Autodesk Fusion 360 part; units mm, degrees
sketch "Sketch1" plane through (0, 0, 0) normal (0, 0, 1) x (1, 0, 0)
  line L0 (0, 0) -> (10, 0)
  line L1 (10, 0) -> (10, 10)
  line L2 (10, 10) -> (0, 10)
  line L3 (0, 10) -> (0, 0)
  line L4 (0, 10) -> (10, 0)
  line L5 (0, 0) -> (10, 10)
  circle A0 centre (5, 5) radius 2
  dimension "d1" = 10
  dimension "d2" = 10
  dimension "d3" = 4
extrude "Extrude1" add sketch "Sketch1" along normal blind 2.5 contours L0 L4 L5 A0 | L3 L4 L5 A0 | L1 L4 L5 A0 | L2 L4 L5 A0
sketch "Sketch2" plane through (0, 0, 2.5) normal (0, 0, 1) x (-1, 0, 0)
  circle A0 centre (-5, -5) radius 2
  line L0 (0, -10) -> (0, 0)
  line L1 (0, 0) -> (-10, 0)
  line L2 (-10, 0) -> (-10, -10)
  line L3 (-10, -10) -> (0, -10)
  line L4 (0, 0) -> (-10, 0)
  line L5 (-10, 0) -> (-10, 2)
  line L6 (-10, 2) -> (0, 2)
  line L7 (0, 2) -> (0, 0)
  line L8 (0, 0) -> (-10, 0)
  line L9 (-10, 0) -> (-10, 1.5)
  line L10 (-10, 1.5) -> (0, 1.5)
  line L11 (0, 1.5) -> (0, 0)
  line L12 (-5, 0) -> (3, 0)
  line L13 (3, 0) -> (3, 1.5)
  line L14 (3, 1.5) -> (-5, 1.5)
  line L15 (-5, 1.5) -> (-5, 0)
  line L16 (-5, 0) -> (-13, 0)
  line L17 (-13, 0) -> (-13, 1.5)
  line L18 (-13, 1.5) -> (-5, 1.5)
  line L19 (-5, 1.5) -> (-5, 0)
  line L20 (3, 0) -> (1.5, 0)
  line L21 (1.5, 0) -> (1.5, 1.5)
  line L22 (1.5, 1.5) -> (3, 1.5)
  line L23 (3, 1.5) -> (3, 0)
  line L24 (3, 0) -> (1.5, 0)
  line L25 (1.5, 0) -> (1.5, 20)
  line L26 (1.5, 20) -> (3, 20)
  line L27 (3, 20) -> (3, 0)
  line L28 (-13, 0) -> (-11.5, 0)
  line L29 (-11.5, 0) -> (-11.5, 20)
  line L30 (-11.5, 20) -> (-13, 20)
  line L31 (-13, 20) -> (-13, 0)
  line L32 (1.5, 20) -> (0, 20)
  line L33 (0, 20) -> (0, 18.5)
  line L34 (0, 18.5) -> (1.5, 18.5)
  line L35 (1.5, 18.5) -> (1.5, 20)
  line L36 (-11.5, 20) -> (-10, 20)
  line L37 (-10, 20) -> (-10, 18.5)
  line L38 (-10, 18.5) -> (-11.5, 18.5)
  line L39 (-11.5, 18.5) -> (-11.5, 20)
  line L40 (1.5, 2) -> (-11.5, 2)
  line L41 (-11.5, 2) -> (-11.5, 18.5)
  line L42 (-11.5, 18.5) -> (1.5, 18.5)
  line L43 (1.5, 18.5) -> (1.5, 2)
  line L44 (1.5, 0) -> (0, -1.5)
  line L45 (1.5, 0) -> (3.6213, 0) construction
  line L46 (-11.5, 0) -> (-10, -1.5)
  dimension "d6" = 2
  dimension "d7" = 1.5
  dimension "d8" = 8
  dimension "d9" = 20
  dimension "d10" = 1.5
  dimension "d11" = 20
  dimension "d12" = 1.5
  dimension "d13" = 1.5
  dimension "d14" = 1.5
  dimension "d15" = 1.5
  dimension "d16" = 135
  dimension "d17" = 90
extrude "Extrude2" add sketch "Sketch2" along normal blind 2 contours L0 L1 L2 L3 L4 L8 L12 L16 | L0 L12 L44 | L1 L4 L7 L8 L10 L11 L12 L14 L15 L19 | L7 L11 L12 L14 L21 L25 | L2 L16 L46 | L1 L4 L5 L8 L9 L10 L15 L16 L18 L19 | L5 L6 L7 L10 L14 L18 L40 | L7 L14 L25 L40 | L5 L9 L16 L18 L29 | L6 L25 L29 L34 L38 L40 L41 L42 L43 | L5 L18 L29 L40
sketch "Sketch3" plane through (0, 0, 2.5) normal (0, 0, -1) x (1, 0, 0)
  line L0 (10, 0) -> (10, -1.5)
  line L1 (10, -1.5) -> (11.5, 0)
  line L2 (11.5, 0) -> (11.5, 18.5)
  line L3 (11.5, 18.5) -> (-1.5, 18.5)
  line L4 (-1.5, 18.5) -> (-1.5, 0)
  line L5 (-1.5, 0) -> (0, -1.5)
  line L6 (0, -1.5) -> (0, 0)
  line L7 (0, 0) -> (10, 0)
  line L8 (-1.5, 0) -> (11.5, 0)
  line L9 (11.5, 0) -> (11.5, -1.5)
  line L10 (11.5, -1.5) -> (-1.5, -1.5)
  line L11 (-1.5, -1.5) -> (-1.5, 0)
  line L12 (-1.5, 0) -> (11.5, 0)
  line L13 (11.5, 0) -> (11.5, 2)
  line L14 (11.5, 2) -> (-1.5, 2)
  line L15 (-1.5, 2) -> (-1.5, 0)
  line L16 (-1.5, 18.5) -> (-1, 18.5)
  line L17 (-1, 2) -> (-1.5, 2)
  line L18 (-1.5, 2) -> (-1.5, 18.5)
  line L19 (11.5, 18.5) -> (11, 18.5)
  line L20 (11, 2) -> (11.5, 2)
  line L21 (11.5, 2) -> (11.5, 18.5)
  line L22 (-1.5, 18.5) -> (0, 18.5)
  line L23 (0, 18.5) -> (0, 20)
  line L24 (0, 20) -> (-1.5, 20)
  line L25 (-1.5, 20) -> (-1.5, 18.5)
  line L26 (11.5, 18.5) -> (10, 18.5)
  line L27 (10, 18.5) -> (10, 20)
  line L28 (10, 20) -> (11.5, 20)
  line L29 (11.5, 20) -> (11.5, 18.5)
  line L30 (10, 20) -> (9.75, 20)
  line L31 (9.75, 20) -> (9.75, 18.5)
  line L32 (9.75, 18.5) -> (10, 18.5)
  line L33 (10, 18.5) -> (10, 20)
  line L34 (0, 20) -> (0.25, 20)
  line L35 (0.25, 20) -> (0.25, 18.5)
  line L36 (0.25, 18.5) -> (0, 18.5)
  line L37 (0, 18.5) -> (0, 20)
  line L38 (-1.5, 20) -> (-1.25, 20)
  line L39 (-1.25, 20) -> (-1.25, 2)
  line L40 (-1.25, 2) -> (-1.5, 2)
  line L41 (-1.5, 2) -> (-1.5, 20)
  line L42 (11.5, 2) -> (11.25, 2)
  line L43 (11.25, 2) -> (11.25, 18.5)
  line L44 (11.25, 18.5) -> (11.5, 18.5)
  line L45 (11.5, 18.5) -> (11.5, 2)
  line L46 (-1.5, 18.5) -> (0.25, 18.5)
  line L47 (0.25, 18.5) -> (0.25, 18.25)
  line L48 (0.25, 18.25) -> (-1.5, 18.25)
  line L49 (-1.5, 18.25) -> (-1.5, 18.5)
  line L50 (9.75, 18.5) -> (11.25, 18.5)
  line L51 (11.25, 18.5) -> (11.25, 18.25)
  line L52 (11.25, 18.25) -> (9.75, 18.25)
  line L53 (9.75, 18.25) -> (9.75, 18.5)
  line L54 (0.25, 20) -> (9.75, 20)
  line L55 (9.75, 20) -> (9.75, 18.5)
  line L56 (9.75, 18.5) -> (0.25, 18.5)
  line L57 (0.25, 18.5) -> (0.25, 20)
  dimension "d20" = 13
  dimension "d21" = 2
  dimension "d22" = 0.5
  dimension "d23" = 0.5
  dimension "d24" = 1.5
  dimension "d25" = 1.5
  dimension "d26" = 1.5
  dimension "d27" = 1.5
  dimension "d28" = 0.25
  dimension "d29" = 0.25
  dimension "d30" = 0.25
  dimension "d31" = 0.25
  dimension "d32" = 0.25
  dimension "d33" = 0.25
extrude "Extrude3" add sketch "Sketch3" along normal blind 1 contours L3 L14 L17 L20 L39 L43 L47 L48 L52 L53 L56 | L3 L31 L35 L54 L55 L56 L57
sketch "Sketch4" plane through (0, 0, 1.5) normal (0, 0, -1) x (1, 0, 0)
  line L0 (0.25, 18.25) -> (-1.25, 18.25)
  line L1 (-1.25, 18.25) -> (-1.25, 2)
  line L2 (-1.25, 2) -> (11.25, 2)
  line L3 (11.25, 2) -> (11.25, 18.25)
  line L4 (11.25, 18.25) -> (9.75, 18.25)
  line L5 (9.75, 18.25) -> (9.75, 20)
  line L6 (9.75, 20) -> (0.25, 20)
  line L7 (0.25, 20) -> (0.25, 18.25)
  line L8 (0.25, 20) -> (9.75, 20)
  line L9 (9.75, 20) -> (9.75, 18.5)
  line L10 (9.75, 18.5) -> (0.25, 18.5)
  line L11 (0.25, 18.5) -> (0.25, 20)
  dimension "d36" = 1.5
extrude "Extrude4" add sketch "Sketch4" along normal blind 0.5 contours L5 L6 L7 L8 L9 L10 L11
extrude "Extrude5" add 1 faces at (3.4167, -19, 2.5) along direction (0, 0, 1) blind 2
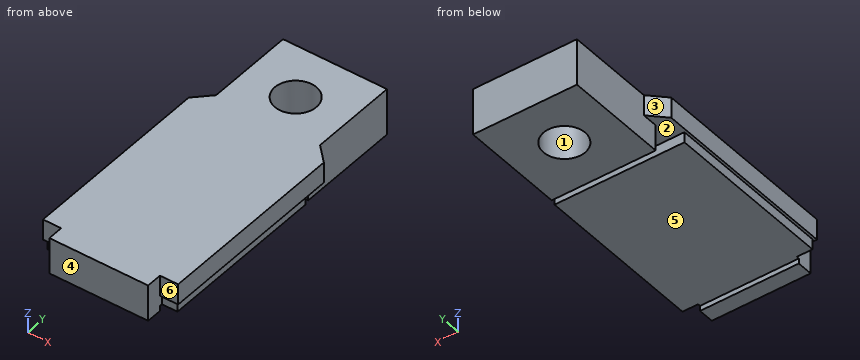
The listing builds one solid part. Answer for the finished solid, in the listing's coordinates (mm). Face numbers are marked on the shaded views. A direction names the side the tool comes from. Round coordinates to 2 decimals unless told otherwise and drop trailing zeros. Write each loop counter-clockwise with the first axis right and the second up, starting at its lowest first coordinate (ties: lowest second). Pieces come first, ordered by that corner, then holes. Notation, with made-up numbers: (-31, 28.25) - (21, 28.25) arc R32 ccw to (21, 54.25) - close; hole circle Ø6 at (10, -15.5). An arc over 180 degrees is marked (long way). Use a Markdown table: item, result. Add a question column.
1. Consider line 1 (Y direction, x = 5, z = 1.4); line 2 (Y direction, x = 5, z = 1.85); line 3 (X direction, y = 5, z = 2.65). Determine where each line is inside the solid, lowest interval first.
2. The part is cut by section A-A (z = 1.95). Write down the section's boundary in (x, y), and give its area (3 significant figures).
3. The part is cut by section B-B (x = 9). Write down the section's boundary in (y, z), and give its area (3 significant figures).
4. A tool of negligible diameter and unlimited length cuts with its end or side. For the marked faces 4, 5 and 6, from which of +Z, -Z, +X, -X, +Y, -Y can it reach the whole face along a straight path? Write none if from no direction.
5. Flat-ended cylindrical pins translate along their axes: P1, Ø1.5, axis at y = 6.5, z = 1.5, coming from the +X side; P2, Ø6.5, axis at x = 2, y = -12.5, coming from the -Z side; P3, Ø0.8, axis at x = 6.5, y = -19.5, coming from the -Z side; P4, Ø0.9, axis at x = 0, z = 4, coming from the -Y side. Find the tip coordinate at first contact, or state that the pin passes through.
6. For a pull along X with two mould halves and no side action, classify the marked faces 1, 2 and 3 as +X half, -X half, draft (parallel to the pull), parting line (faces both ways), or undercut.
7. The part is cut by section C-C (y = -10.75). Write down the section's boundary in (x, z).
Reported:
| question | item | result |
|---|---|---|
| 1 | line 1 | -20 to -18.5, 0 to 3, 7 to 10 |
| 1 | line 2 | -20 to -2, 0 to 3, 7 to 10 |
| 1 | line 3 | 0 to 3, 7 to 10 |
| 2 | outline | (-1.25, -18.25) - (0.25, -18.25) - (0.25, -20) - (9.75, -20) - (9.75, -18.25) - (11.25, -18.25) - (11.25, -2) - (-1.25, -2) - close; (0, 0) - (10, 0) - (10, 10) - (0, 10) - close; hole circle Ø4 at (5, 5) |
| 2 | area | 307 mm^2 |
| 3 | outline | (-20, 1) - (-18.5, 1) - (-18.5, 1.5) - (-2, 1.5) - (-2, 2.5) - (0, 2.5) - (0, 0) - (10, 0) - (10, 4.5) - (-20, 4.5) - close |
| 3 | area | 104 mm^2 |
| 4 | face 4 | +Z, -Z, +X, -X, -Y |
| 4 | face 5 | -Z, +X, -X |
| 4 | face 6 | +Z, -Z, +X, -Y |
| 5 | P1 | x = 10 |
| 5 | P2 | z = 1.5 |
| 5 | P3 | z = 1 |
| 5 | P4 | y = -20 |
| 6 | face 1 | undercut |
| 6 | face 2 | draft |
| 6 | face 3 | -X half |
| 7 | outline | (-1.5, 2.5) - (-1.25, 2.5) - (-1.25, 1.5) - (11.25, 1.5) - (11.25, 2.5) - (11.5, 2.5) - (11.5, 4.5) - (-1.5, 4.5) - close |
